Geometry check sheet. Reference: the model listing, model coordinates, mm. Face numbers are marked on the shaded views. A direction names the side the tool comes from. Round coordinates to 2 decimals unless told otherwise and drop trailing zeros. Order: outer loops, then holes, each group sorted by start corner. A loop starts at its lowest first (then second) coordinate and runs counter-clockwise, first axis right, second up. Notation, with made-up numbers: (-9, 12.5) -> (29, 12.5) arc R28 ccw to (29, 46.5) -> close; hole circle Ø6 at (76, -16). An arc over 180 degrees is marked (long way). Answer as a JSON object with one key per item and string values. Group by question number.
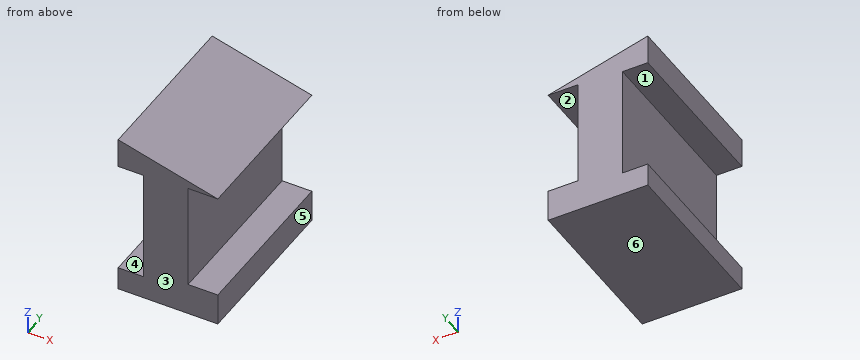
from build123d import *

# Parameters (mm, degrees)
F0_W     = 3.813922
F0_H     = 17.002841
F0_W_2   = 4.474432
F0_H_2   = 16.107955
F1_DEPTH = 25
F2_DEPTH = 25.001
F3_DEPTH = 46


with BuildPart() as f1:
    # F0 (on Front) → F1 (new body)
    with BuildSketch(Plane.XZ):
        Polygon((6.599786, 9.955611), (-8.400214, 13.9826), (-8.400214, 9.508167), (-4.586292, 9.508167), (-4.586292, -7.494674), (-8.400214, -7.494674), (-8.400214, -11.0174), (6.599786, -11.0174), (6.599786, -6.152344), (2.125354, -6.152344), (2.125354, 9.955611), align=None)
        Polygon((6.599786, 13.9826), (-8.400214, 13.9826), (6.599786, 9.955611), align=None)
        with Locations((-6.493253, 1.006747)):
            Rectangle(F0_W, F0_H)
        with Locations((4.36257, 1.901633)):
            Rectangle(F0_W_2, F0_H_2)
    extrude(amount=F1_DEPTH)

    # F0 (on Front) → F2 (cut, through all)
    with BuildSketch(Plane.XZ):
        with Locations((4.36257, 1.901633)):
            Rectangle(F0_W_2, F0_H_2)
        with Locations((-6.493253, 1.006747)):
            Rectangle(F0_W, F0_H)
    extrude(amount=F2_DEPTH, mode=Mode.SUBTRACT)

    # F0 (on Front) → F3 (cut)
    with BuildSketch(Plane.XZ):
        Polygon((6.599786, 13.9826), (-8.400214, 13.9826), (6.599786, 9.955611), align=None)
    extrude(amount=F3_DEPTH, mode=Mode.SUBTRACT)


solid = f1.part
Item 1: Sectioned sample at D-D, the plane z = 7. Enter the section's corners in (x, y).
Item 2: Mould release check, pull along Z, two halves, no side actions. Record for the marked faces 4, 5 and 6: pulls with the +Z half, pulls with the -Z half, needs draft (parallel to the pull), parting line crosses it, or undercut.
Item 3: Sectioned sample at C-C, the plane x = 3. Enter the section's corners in (y, z), then the cut area to 3 significant figures.
Item 4: Thickness scan on L1, parallel to X at y = -10.75, z = 1.25; L2, parallel to Z at x = -6.25, y = -17.5; L3, parallel to Z at x = 4, y = -4.75. Record the ranges inside material, lowest first.
Item 5: Sectioned sample at B-B, the plane y = -14. Enter the section's corners in (x, z).
Item 6: Sectioned sample at A-A, the plane x = -7. Enter the section's corners in (y, z), then the cut area to 3 significant figures.
Item 7: Depth check by flat-ended pin: pin 1 Ø3 at (x, y) = (-6.5, -14.5) entering from +Z; pin 2 Ø12 at (y, z) = (-3.5, -3.5) entering from -X; pin 3 Ø13 at (y, z) = (-17, 1.5) entering from +X; pin 4 Ø3 at (x, y) = (-2, -10.5) entering from +Z. Enter the tip coordinate at first touch or a pass-through.
Item 8: Set-up check for the marked faces 1, 2 and 3: record each of +Z, -Z, +X, -X, +Y, -Y from which the full face is reachable in a straight line by a thin tool's end or side.
Result:
{
 "1": {"outline": "(-4.59, -25) -> (2.13, -25) -> (2.13, 0) -> (-4.59, 0) -> close"},
 "2": {"face 4": "undercut", "face 5": "needs draft", "face 6": "pulls with the -Z half"},
 "3": {"outline": "(-25, -11.02) -> (0, -11.02) -> (0, -6.15) -> (-25, -6.15) -> close; (-25, 9.96) -> (0, 9.96) -> (0, 10.92) -> (-25, 10.92) -> close", "area": "146 mm2"},
 "4": {"L1": "x = -4.59 to 2.13", "L2": "z = -11.02 to -7.49, 9.51 to 13.41", "L3": "z = -11.02 to -6.15, 9.96 to 10.65"},
 "5": {"outline": "(-8.4, -11.02) -> (6.6, -11.02) -> (6.6, -6.15) -> (2.13, -6.15) -> (2.13, 9.96) -> (6.6, 9.96) -> (-8.4, 13.98) -> (-8.4, 9.51) -> (-4.59, 9.51) -> (-4.59, -7.49) -> (-8.4, -7.49) -> close"},
 "6": {"outline": "(-25, -11.02) -> (0, -11.02) -> (0, -7.49) -> (-25, -7.49) -> close; (-25, 9.51) -> (0, 9.51) -> (0, 13.61) -> (-25, 13.61) -> close", "area": "191 mm2"},
 "7": {"pin 1": "stops at z = 13.88", "pin 2": "stops at x = -8.4", "pin 3": "stops at x = 2.13", "pin 4": "stops at z = 12.67"},
 "8": {"face 1": "-X, +Y, -Y", "face 2": "+X, +Y, -Y", "face 3": "+Z, -Z, +X, -X, -Y"}
}
